Can you work these out from the model? Positions are in its coordinate system, mm. Round coordinates to 2 decimals unless told otherwise and drop trailing zeros. Loops run counter-clockwise (first coordinate to the right, second up) from the corner with the lowest first, then second, coordinate; pieces in that order, holes last. Notation, with made-up numbers: M 3,72 L 44,72 A16 cw 44,90 Z; hole C 1,84 d11. An arc over 180 degrees is marked long. Return JSON: item names as keys, results as strings.
```python
from build123d import *

# Parameters (mm, degrees)
SZKIC1_R                    = 6.5
DODANIE_WYCI_GNI_CIE1_DEPTH = 3
ZAOKR_GLENIE1_R             = 0.2


with BuildPart() as part:
    # Szkic1 → Dodanie-wyciągnięcie1 (new body, symmetric)
    with BuildSketch(Plane(origin=(0, 0, 0), x_dir=(1, 0, 0), z_dir=(0, 1, 0))):
        Circle(SZKIC1_R)
    extrude(amount=DODANIE_WYCI_GNI_CIE1_DEPTH, both=True)

    # Szkic3 → Wycięcie-obrót1 (revolve, cut)
    with BuildSketch(Plane.XY):
        with BuildLine():
            Line((0, -5.55), (0, 5.55))
            ThreePointArc((0, 5.55), (5.55, 0), (0, -5.55))
        make_face()
    revolve(axis=Axis((0, -5.55, 0), (0, 1, 0)), mode=Mode.SUBTRACT)

    # Zaokrąglenie1
    zaokr_glenie1_edges = [part.edges().sort_by_distance(p)[0] for p in [
        (-6.5, -3, 0),
        (-6.5, 3, 0),
    ]]
    fillet(zaokr_glenie1_edges, radius=ZAOKR_GLENIE1_R)


solid = part.part
```
Q1. Suppose I cut it at B-B, the plane z = 0. Please give me the cut outline in (x, y), plus the area to 3 significant figures.
Results:
{"outline": "M -6.5,-2.8 A0.2 ccw -6.3,-3 L -4.67,-3 A5.55 cw -4.67,3 L -6.3,3 A0.2 ccw -6.5,2.8 Z; M 4.67,-3 L 6.3,-3 A0.2 ccw 6.5,-2.8 L 6.5,2.8 A0.2 ccw 6.3,3 L 4.67,3 A5.55 cw Z", "area": "14.8 mm2"}
Q2. Suppose I cut it at D-D, the plane y = -2.5. Please give me the cut outline in (x, z), plus the area to 3 significant figures.
Results:
{"outline": "C 0,0 d13; hole C 0,0 d9.91", "area": "55.6 mm2"}
Q3. Suppose I cut it at A-A, the plane x = 0. Please give me the cut outline in (y, z).
Results:
{"outline": "M -3,-6.3 A0.2 ccw -2.8,-6.5 L 2.8,-6.5 A0.2 ccw 3,-6.3 L 3,-4.67 A5.55 cw -3,-4.67 Z; M -3,4.67 A5.55 cw 3,4.67 L 3,6.3 A0.2 ccw 2.8,6.5 L -2.8,6.5 A0.2 ccw -3,6.3 Z"}
Q4. If I drill on line 1 along X through (y, z) = (0.75, -0.25); line 2 along Z through (x, y) = (-2.5, -2.25); line 3 along Z through (x, y) = (-2, 2.25), over which ranges is the centre line in solid material (lowest first)?
Results:
{"line 1": "x = -6.5 to -5.49, 5.49 to 6.5", "line 2": "z = -6 to -4.41, 4.41 to 6", "line 3": "z = -6.18 to -4.66, 4.66 to 6.18"}
Q5. I'm going to push flat-ended pins straight in: pin 1 Ø4 at (x, z) = (3.5, -2.5) entering from +Y; pin 2 Ø1 at (x, y) = (5, 1) entering from +Z; pin 3 Ø2 at (x, y) = (1.5, -2) entering from +Z. Where does each tip first touch, or does it pass through?
Results:
{"pin 1": "stops at y = 3", "pin 2": "stops at z = 4.69", "pin 3": "stops at z = 6.48"}
Q6. Suppose I cut it at C-C, the plane y = 0.5. Please give me the cut outline in (x, z), plus the area to 3 significant figures.
Results:
{"outline": "C 0,0 d13; hole C 0,0 d11.05", "area": "36.7 mm2"}
